Geometry: final body of the model. Coordinates: model frame, mm. Face numbers are marked on the shaded views. A direction names the side the tool comes from. Coordinates: 2 decimals unless noted, no trailing zeros. Order: outer loops, then holes, each group sorted by start corner. A loop starts at its lowest first (then second) coordinate and runs counter-clockwise, first axis right, second up. Notation, with made-up numbers: M 39,33 L 49,33 A10 ccw 49,52 Z; hole C -17,42 d3. An arc over 180 degrees is marked long. One line per question, with ' | ' between items.
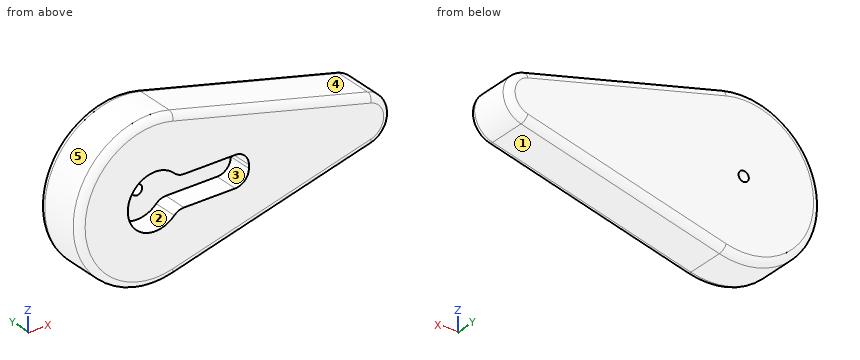
from build123d import *

# Parameters (mm, degrees)
SKETCH1_R               = 1.5
CAM_DEPTH               = 15
CAM_FILLET_2MM_R        = 2
SERVO_ADAPTER_CUT_DEPTH = 7
FILLET_4_5MM_R          = 4


with BuildPart() as part:
    # Sketch1 → Cam (new body)
    with BuildSketch(Plane(origin=(0, 0, 0), x_dir=(1, 0, 0), z_dir=(0, 1, 0))):
        with BuildLine():
            ThreePointArc((5.625, 21.785531322), (-22.5, 0), (5.625, -21.785531322))
            Line((5.625, -21.785531322), (63.75, -6.777720856))
            ThreePointArc((63.75, -6.777720856), (69, 0), (63.75, 6.777720856))
            Line((63.75, 6.777720856), (5.625, 21.785531322))
        make_face()
        with Locations(Location((0, 0, 0), (0, 0, 270))):
            Circle(SKETCH1_R, mode=Mode.SUBTRACT)
    extrude(amount=CAM_DEPTH)

    # Cam_Fillet_2mm
    cam_fillet_2mm_edges = [part.edges().sort_by_distance(p)[0] for p in [
        (34.6875, 15, -14.281626089),
        (-22.5, 15, 0),
        (34.6875, 15, 14.281626089),
        (69, 15, 0),
        (34.6875, 0, 14.281626089),
        (-22.5, 0, 0),
        (34.6875, 0, -14.281626089),
        (69, 0, 0),
    ]]
    fillet(cam_fillet_2mm_edges, radius=CAM_FILLET_2MM_R)

    # Sketch2 → Servo_adapter_cut (cut)
    with BuildSketch(Plane.XZ):
        with BuildLine():
            Line((0, 1.5), (0, 4.5))
            Line((0, 4.5), (6.614378278, 4.5))
            ThreePointArc((6.614378278, 4.5), (-8, 0), (6.614378278, -4.5))
            Line((6.614378278, -4.5), (0, -4.5))
            Line((0, -4.5), (0, -1.5))
            ThreePointArc((0, -1.5), (-1.5, 0), (0, 1.5))
        make_face()
        with BuildLine():
            Line((6.614378278, 4.5), (0, 4.5))
            Line((0, 4.5), (0, 1.5))
            ThreePointArc((0, 1.5), (1.060660172, 1.060660172), (1.5, 0))
            ThreePointArc((1.5, 0), (1.060660172, -1.060660172), (0, -1.5))
            Line((0, -1.5), (0, -4.5))
            Line((0, -4.5), (6.614378278, -4.5))
            ThreePointArc((6.614378278, -4.5), (7.645751311, -2.354248689), (8, 0))
            ThreePointArc((8, 0), (7.645751311, 2.354248689), (6.614378278, 4.5))
        make_face()
        with BuildLine():
            Line((27.5, 4.5), (6.614378278, 4.5))
            ThreePointArc((6.614378278, 4.5), (7.645751311, 2.354248689), (8, 0))
            ThreePointArc((8, 0), (7.645751311, -2.354248689), (6.614378278, -4.5))
            Line((6.614378278, -4.5), (27.5, -4.5))
            Line((27.5, -4.5), (27.5, 4.5))
        make_face()
    extrude(amount=-SERVO_ADAPTER_CUT_DEPTH, mode=Mode.SUBTRACT)

    # Fillet_4.5mm
    fillet_4_5mm_edges = [part.edges().sort_by_distance(p)[0] for p in [
        (6.614378278, 3.5, -4.5),
        (6.614378278, 3.5, 4.5),
        (27.5, 3.5, 4.5),
        (27.5, 3.5, -4.5),
    ]]
    fillet(fillet_4_5mm_edges, radius=FILLET_4_5MM_R)


solid = part.part
1. Section A-A, the plane y = 5.5. Output: boundary loops of the cut face in (x, z) (3 decimals).
Response values:
outline: M 5.625,-21.786 L 63.75,-6.778 A7 ccw 63.75,6.778 L 5.625,21.786 A22.5 ccw long Z; hole M 5.647,-5.667 A4 cw 8.471,-4.5 L 23.5,-4.5 A4 ccw 27.5,-0.5 L 27.5,0.5 A4 ccw 23.5,4.5 L 8.471,4.5 A4 cw 5.647,5.667 A8 ccw long Z
2. Pin query (flat end, axial travel): P1, Ø7.5, axis at x = 17.5, y = 5, coming from the -Z side; P2, Ø5, axis at x = 36.5, y = 7.5, coming from the +Z side; P3, Ø1.5, axis at y = 9, z = 6, coming from the +X side. Return the tip coordinate at first contact, or that it passes through.
Response values:
P1: stops at z = -19.69 | P2: stops at z = 14.46 | P3: stops at x = 66.63
3. Draft query along Z for the marked faces 3, 4 and 5. Return one class per face: pulls with the +Z half, pulls with the -Z half, needs draft (parallel to the pull), parting line crosses it, or undercut.
Response values:
face 3: undercut | face 4: pulls with the +Z half | face 5: parting line crosses it
4. Access query for the marked faces 1 and 2. Directions: +Z, -Z, +X, -X, +Y, -Y. A direction counts if a zero-diameter tool reaches every point of the face in a straight line with its end or side. Return the directions, or none.
Response values:
face 1: -Z, +X, +Y, -Y | face 2: -Y
5. Material intervals for line 1 (Z direction, x = 0, y = 10.25); line 2 (Z direction, x = 0, y = 5); line 3 (X direction, y = 5.5, z = 3.5), sorted ascending. Write a range as [from, to].
Response values:
line 1: z = [-22.5, -1.5], [1.5, 22.5] | line 2: z = [-22.5, -8], [8, 22.5] | line 3: x = [-22.23, -7.19], [26.15, 68.06]
